For this review, take the finished solid that the model builds, in its own axes (mm). A direction names the side the tool comes from. Give positions to 0.01 mm unless a question says otherwise; leave off trailing zeros. Write each loop counter-clockwise with the first axis right and the second up, starting at its lowest first coordinate (ties: lowest second). Pieces come first, ordered by that corner, then holes. Notation, with made-up numbers: M -5.75,-11.75 L 47.25,-11.75 A12 cw 47.25,-4.75 Z; hole C -36.75,52.5 d1. An arc over 180 degrees is marked long. One line per item, written item: value. Start each with the question number.
Item 1: To check wall thickness, follow probe 1 along X at (y, z) = (117, -31.29); probe 2 along X at (y, z) = (114, -31); probe 3 along Z at (x, y) = (71.93, 112.25). State the ranges of each line that lie inside material, in increasing order.
Item 2: Clearance check with flat-ended pins moving along their axes: pin 1 Ø0.9 at (x, z) = (72, -31) entering from +Y; pin 2 Ø8 at (x, z) = (38, -20.5) entering from +Y; pin 3 Ø6 at (x, y) = (12.5, 48) entering from -Z. State where each tip first meets the part, or that it passes through.
Item 3: Consider section A-A, the plane x = 26. Write out the cut boundary in (y, z) (3 decimals).
Item 4: Consider section B-B, the plane y = 105.5. Write out the cut boundary in (x, z).
Item 5: Consider section D-D, the plane y = 52. Write out the cut boundary in (x, z).
Item 6: Mouldability with a two-part tool opening along Z and no side actions: class faces 1 (the face through (67, 87, -22.21)), 2 (the face through (37, 43, -2.54)), 3 (the face through (0.86, 0.9, -18.86)) as released by +Z, released by -Z, zero draft, split by the parting line, or undercut.
Item 7: Consider section C-C, the plane z = -19. Write out the cut boundary in (x, y), and give its area (3 significant figures).
Item 8: Tool access review of faces 4 (the face through (36.98, 0.9, -0.86)), 5 (the face through (2.54, 43, -18)), 6 (the face through (37, 105, -29.21)): name each direction out of +Z, -Z, +X, -X, +Y, -Y from which nothing blocks a thin tool from reaching the whole face with its end or side.
```python
from build123d import *

# Parameters (mm, degrees)
SKETCH1_W           = 74.93
SKETCH1_H           = 34.29
BOSS_EXTRUDE1_DEPTH = 87.122
SHELL1_T            = -2.54
SKETCH12_W          = 74.93
SKETCH12_H          = 34.29
BOSS_EXTRUDE6_DEPTH = 34.29
SHELL2_T            = -5.08
CUT_EXTRUDE13_REACH = 123.777
SKETCH18_W          = 12.7
SKETCH18_H          = 9.525
SKETCH18_W_2        = 5
SKETCH18_H_2        = 10.13
SKETCH20_R          = 1.5
CUT_EXTRUDE14_DEPTH = 20
FILLET1_R           = 3


with BuildPart() as part:
    # Sketch1 → Boss-Extrude1 (new body)
    with BuildSketch(Plane(origin=(0, 0, 0), x_dir=(1, 0, 0), z_dir=(0, 1, 0))):
        with Locations((37.465, 17.145)):
            Rectangle(SKETCH1_W, SKETCH1_H)
    extrude(amount=BOSS_EXTRUDE1_DEPTH)

    # Shell1
    shell1_openings = [part.faces().sort_by_distance(p)[0] for p in [
        (37.465, 43.561, -34.29),
    ]]
    offset(amount=SHELL1_T, openings=shell1_openings, kind=Kind.INTERSECTION)

    # Sketch12 → Boss-Extrude6 (add)
    with BuildSketch(Plane(origin=(0, 87.122, 0), x_dir=(1, 0, 0), z_dir=(0, 1, 0))):
        with Locations((37.465, 17.145)):
            Rectangle(SKETCH12_W, SKETCH12_H)
    extrude(amount=BOSS_EXTRUDE6_DEPTH)

    # Shell2
    shell2_openings = [part.faces().sort_by_distance(p)[0] for p in [
        (37.465, 121.412, -17.145),
    ]]
    offset(amount=SHELL2_T, openings=shell2_openings)

    # Sketch18 → Cut-Extrude13 (cut, up to next)
    with BuildSketch(Plane(origin=(0, 89.662, 0), x_dir=(1, 0, 0), z_dir=(0, 1, 0)), mode=Mode.PRIVATE) as cut_extrude13_sk1:
        with Locations((28.575, 9.8425)):
            Rectangle(SKETCH18_W, SKETCH18_H)
    cut_extrude13_tool1 = extrude(cut_extrude13_sk1.sketch, amount=-CUT_EXTRUDE13_REACH, mode=Mode.PRIVATE) & part.part
    # Sketch18 → Cut-Extrude13 (cut, up to next)
    with BuildSketch(Plane(origin=(0, 89.662, 0), x_dir=(1, 0, 0), z_dir=(0, 1, 0)), mode=Mode.PRIVATE) as cut_extrude13_sk2:
        with Locations((67.35, 17.145)):
            Rectangle(SKETCH18_W_2, SKETCH18_H_2)
    cut_extrude13_tool2 = extrude(cut_extrude13_sk2.sketch, amount=-CUT_EXTRUDE13_REACH, mode=Mode.PRIVATE) & part.part
    add(cut_extrude13_tool1.solids().sort_by_distance((28.575, 89.662, -9.8425))[0], mode=Mode.SUBTRACT)
    add(cut_extrude13_tool2.solids().sort_by_distance((67.35, 89.662, -17.145))[0], mode=Mode.SUBTRACT)

    # Sketch20 → Cut-Extrude14 (cut)
    with BuildSketch(Plane(origin=(0, 121.412, 0), x_dir=(1, 0, 0), z_dir=(0, 1, 0))):
        with Locations(Location((3, 31.29, 0), (0, 0, 270))):
            Circle(SKETCH20_R)
        with Locations(Location((3, 3, 0), (0, 0, 270))):
            Circle(SKETCH20_R)
        with Locations(Location((71.93, 3, 0), (0, 0, 270))):
            Circle(SKETCH20_R)
        with Locations(Location((71.93, 31.29, 0), (0, 0, 270))):
            Circle(SKETCH20_R)
    extrude(amount=-CUT_EXTRUDE14_DEPTH, mode=Mode.SUBTRACT)

    # Fillet1
    # the kernel refuses this fillet: 3 mm, written as the material it takes off along each edge
    with BuildSketch(Plane(origin=(71.93, 3, -3), x_dir=(1, 0, 0), z_dir=(0, 0, 1))) as fillet1_piece_1_section:
        Polygon((0, 0), (FILLET1_R, 0), (FILLET1_R, -FILLET1_R), (0, -FILLET1_R), align=None)
    fillet1_piece_1 = extrude(amount=FILLET1_R, mode=Mode.PRIVATE)
    fillet1_piece_1 = fillet1_piece_1 - Plane(origin=(71.93, 3, -3), x_dir=(-0.7071067811865475, 0.7071067811865475, 0), z_dir=(0, 0, 1)) * Sphere(FILLET1_R, mode=Mode.PRIVATE)
    add(fillet1_piece_1, mode=Mode.SUBTRACT)
    with BuildSketch(Plane(origin=(3, 3, -3), x_dir=(-1, 0, 0), z_dir=(0, 0, 1))) as fillet1_piece_2_section:
        Polygon((0, 0), (FILLET1_R, 0), (FILLET1_R, FILLET1_R), (0, FILLET1_R), align=None)
    fillet1_piece_2 = extrude(amount=FILLET1_R, mode=Mode.PRIVATE)
    fillet1_piece_2 = fillet1_piece_2 - Plane(origin=(3, 3, -3), x_dir=(0.7071067811865475, 0.7071067811865475, 0), z_dir=(0, 0, 1)) * Sphere(FILLET1_R, mode=Mode.PRIVATE)
    add(fillet1_piece_2, mode=Mode.SUBTRACT)
    with BuildSketch(Plane(origin=(74.93, 0, -3), x_dir=(0, 1, 0), z_dir=(0, 0, -1)), Plane(origin=(0, 0, -41.79), x_dir=(0, 1, 0), z_dir=(0, 0, 1))) as fillet1_piece_3:
        with BuildLine():
            CenterArc((FILLET1_R, -FILLET1_R), FILLET1_R, 90, 90)
            Line((0, -FILLET1_R), (0, 0))
            Line((0, 0), (FILLET1_R, 0))
        make_face()
    extrude(amount=38.79, mode=Mode.SUBTRACT)
    with BuildSketch(Plane(origin=(3, 0, 0), x_dir=(0, 1, 0), z_dir=(1, 0, 0))) as fillet1_piece_4:
        with BuildLine():
            CenterArc((FILLET1_R, -FILLET1_R), FILLET1_R, 90, 90)
            Line((0, -FILLET1_R), (0, 0))
            Line((0, 0), (FILLET1_R, 0))
        make_face()
    extrude(amount=68.93, mode=Mode.SUBTRACT)
    with BuildSketch(Plane(origin=(74.93, -7.5, -34.29), x_dir=(0, 0, 1), z_dir=(0, 1, 0)), Plane(origin=(0, 128.912, -34.29), x_dir=(0, 0, 1), z_dir=(0, -1, 0))) as fillet1_piece_5:
        with BuildLine():
            CenterArc((FILLET1_R, -FILLET1_R), FILLET1_R, 90, 90)
            Line((0, -FILLET1_R), (0, 0))
            Line((0, 0), (FILLET1_R, 0))
        make_face()
    extrude(amount=136.412, mode=Mode.SUBTRACT)
    with BuildSketch(Plane(origin=(74.93, 3, 0), x_dir=(-1, 0, 0), z_dir=(0, 1, 0)), Plane(origin=(0, 128.912, 0), x_dir=(1, 0, 0), z_dir=(0, -1, 0))) as fillet1_piece_6:
        with BuildLine():
            CenterArc((FILLET1_R, -FILLET1_R), FILLET1_R, 90, 90)
            Line((0, -FILLET1_R), (0, 0))
            Line((0, 0), (FILLET1_R, 0))
        make_face()
    extrude(amount=125.912, mode=Mode.SUBTRACT)


solid = part.part
```
Model answer:
1. probe 1: x = 0 to 1.5, 4.5 to 70.43, 73.43 to 74.93
1. probe 2: x = 0 to 1.53, 4.47 to 70.46, 73.4 to 74.93
1. probe 3: z = -34.29 to -32.79, -29.79 to -4.5, -1.5 to 0
2. pin 1: stops at y = 101.41
2. pin 2: stops at y = 89.66
2. pin 3: stops at z = -2.54
3. outline: M 0,-34.29 L 2.54,-34.29 L 2.54,-2.54 L 84.582,-2.54 L 84.582,-5.08 L 121.412,-5.08 L 121.412,0 L 3,0 A3 ccw 0,-3 Z; M 84.582,-34.29 L 121.412,-34.29 L 121.412,-29.21 L 89.662,-29.21 L 89.662,-14.605 L 84.582,-14.605 Z
4. outline: M 0,-31.29 A3 ccw 3,-34.29 L 71.93,-34.29 A3 ccw 74.93,-31.29 L 74.93,-3 A3 ccw 71.93,0 L 3,0 A3 ccw 0,-3 Z; hole C 3,-31.29 d3; hole C 3,-3 d3; hole M 5.08,-29.21 L 69.85,-29.21 L 69.85,-5.08 L 5.08,-5.08 Z; hole C 71.93,-31.29 d3; hole C 71.93,-3 d3
5. outline: M 0,-31.29 A3 ccw 2.54,-34.25 L 2.54,-2.54 L 72.39,-2.54 L 72.39,-34.25 A3 ccw 74.93,-31.29 L 74.93,-3 A3 ccw 71.93,0 L 3,0 A3 ccw 0,-3 Z
6. face 1: undercut
6. face 2: released by -Z
6. face 3: zero draft
7. outline: M 0,3 A3 ccw 3,0 L 71.93,0 A3 ccw 74.93,3 L 74.93,121.41 L 69.85,121.41 L 69.85,84.58 L 72.39,84.58 L 72.39,2.54 L 2.54,2.54 L 2.54,84.58 L 64.85,84.58 L 64.85,89.66 L 5.08,89.66 L 5.08,121.41 L 0,121.41 Z
7. area: 1,280 mm2
8. face 4: +Z, +X, -X, -Y
8. face 5: -Z
8. face 6: +Y
